Could you check a few things on this drawing? It's one solid part, dimensions in mm from its lowest x, y, z. A direction names the side the tool comes from. Coordinates: 2 decimals unless noted, no trailing zeros. Write each loop counter-clockwise with the first axis right and the second up, starting at its lowest first coordinate (ties: lowest second). Pieces come first, ordered by that corner, then holes.
Item 1: I want a section at B-B (y = 37). Please give me the cut outline in (x, z).
Item 2: I'm going to push a flat-ended pin straight in: P1, Ø12, axis at x = 29.5, y = 35, coming from the -Z side. Where does the tip first touch, or does it pass through?
Item 3: If we mould it in two halves opening along X, with no side actions, what happens to the marked faces 3, 4 and 5? For each: pulls with the +X half, pulls with the -X half, needs draft (parallel to the pull), parting line crosses it, or undercut.
Item 4: I want a section at C-C (x = 61.5). Please give me the cut outline in (y, z).
Item 5: Please list where these lines run through material, in increasing order: line 1 (X direction, y = 18, z = 27.5); line 2 (Z direction, x = 15.5, y = 34).
Item 6: For the marked faces 1 and 2, which set-ups out of +Z, -Z, +X, -X, +Y, -Y let a thin tool reach every point of the face, with its end or its side?
Item 7: I want a section at A-A (z = 28.5). Please give me the cut outline in (x, y).
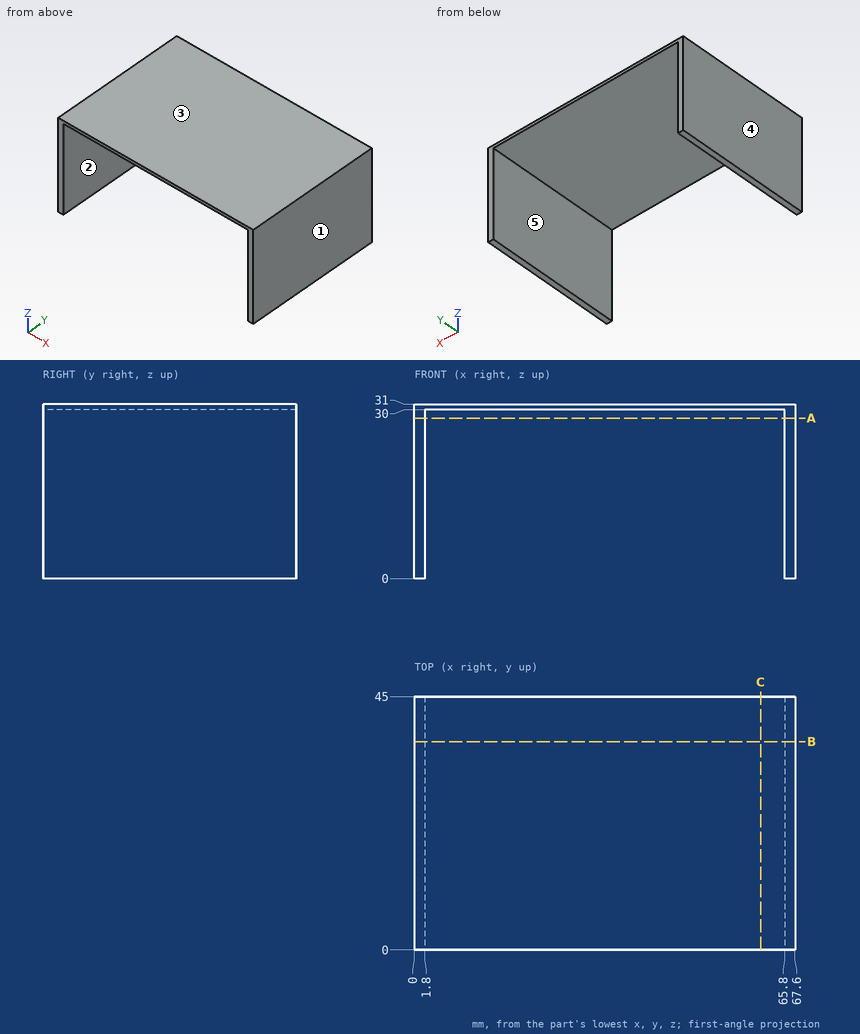
Answer:
1. outline: (0, 0) - (1.8, 0) - (1.8, 30) - (65.8, 30) - (65.8, 0) - (67.6, 0) - (67.6, 31) - (0, 31) - close
2. P1: stops at z = 30
3. face 3: needs draft
3. face 4: pulls with the -X half
3. face 5: undercut
4. outline: (0, 30) - (45, 30) - (45, 31) - (0, 31) - close
5. line 1: x = 0 to 1.8, 65.8 to 67.6
5. line 2: z = 30 to 31
6. face 1: +Z, -Z, +X, +Y, -Y
6. face 2: -Z, +Y, -Y
7. outline: (0, 0) - (1.8, 0) - (1.8, 45) - (0, 45) - close; (65.8, 0) - (67.6, 0) - (67.6, 45) - (65.8, 45) - close
